```python
from build123d import *

# Parameters (mm, degrees)
F0_R     = 26
F0_R_2   = 14
F1_DEPTH = 12
F2_DEPTH = 178
F3_SIZE  = 2
F4_R     = 2.5
F5_DEPTH = 12
F7_DEPTH = 45
F8_R     = 5
F9_DEPTH = 22


with BuildPart() as f1:
    # F0 (on Right) → F1 (new body)
    with BuildSketch(Plane.YZ):
        Circle(F0_R)
        Circle(F0_R_2, mode=Mode.SUBTRACT)
        Circle(F0_R_2)
    extrude(amount=F1_DEPTH)

    # F0 (on Right) → F2 (join)
    with BuildSketch(Plane.YZ):
        Circle(F0_R_2)
    extrude(amount=F2_DEPTH)

    # F3
    f3_edges = [f1.edges().sort_by_distance(p)[0] for p in [
        (0, -26, 0),
        (178, -14, 0),
    ]]
    chamfer(f3_edges, length=F3_SIZE)

    # F4 (on face) → F5 (cut, through all)
    with BuildSketch(Plane(origin=(0, 0, 0), x_dir=(0, -1, 0), z_dir=(-1, 0, 0))):
        with Locations((21, 0)):
            Circle(F4_R)
    extrude(amount=-F5_DEPTH, mode=Mode.SUBTRACT)

    # F6 (on face) → F7 (cut)
    with BuildSketch(Plane.YZ.offset(178)):
        with BuildLine():
            Line((-11, 4.7958315233), (-11, 8.6602540378))
            ThreePointArc((-11, 8.6602540378), (-14, 0), (-11, -8.6602540378))
            Line((-11, -8.6602540378), (-11, -4.7958315233))
            ThreePointArc((-11, -4.7958315233), (-12, 0), (-11, 4.7958315233))
        make_face()
        with BuildLine():
            Line((-11, -4.7958315233), (-11, 4.7958315233))
            ThreePointArc((-11, 4.7958315233), (-12, 0), (-11, -4.7958315233))
        make_face()
        with BuildLine():
            ThreePointArc((12, 0), (11.7473401245, 2.4494897428), (11, 4.7958315233))
            Line((11, 4.7958315233), (11, -4.7958315233))
            ThreePointArc((11, -4.7958315233), (11.7473401245, -2.4494897428), (12, 0))
        make_face()
        with BuildLine():
            ThreePointArc((11, -8.6602540378), (13.2287565553, -4.582575695), (14, 0))
            ThreePointArc((14, 0), (13.2287565553, 4.582575695), (11, 8.6602540378))
            Line((11, 8.6602540378), (11, 4.7958315233))
            ThreePointArc((11, 4.7958315233), (11.7473401245, 2.4494897428), (12, 0))
            ThreePointArc((12, 0), (11.7473401245, -2.4494897428), (11, -4.7958315233))
            Line((11, -4.7958315233), (11, -8.6602540378))
        make_face()
    extrude(amount=-F7_DEPTH, mode=Mode.SUBTRACT)

    # F8 (on face) → F9 (cut, through all)
    with BuildSketch(Plane.XZ.offset(11)):
        with Locations((158, 0)):
            Circle(F8_R)
    extrude(amount=-F9_DEPTH, mode=Mode.SUBTRACT)


solid = f1.part
```
Source: CAD feature listing. Evaluate the final solid. Frame: model axes, mm. A direction names the side the tool comes from. Coordinates: 2 decimals unless noted, no trailing zeros. Loops run counter-clockwise (first coordinate to the right, second up) from the corner with the lowest first, then second, coordinate; pieces in that order, holes last. Notation, with made-up numbers: M 34,52 L 41,52 A34 ccw 41,88 Z; hole C 14.5,65 d7. An arc over 180 degrees is marked long. Use a Markdown table: item, result. Add a question column.
Q1. Material intervals for L1, parallel to X at y = -14.5, z = 16; L2, parallel to Z at x = 158, y = 5.25; L3, parallel to Y at x = 146, z = -1.5, sorted ascending.
Q2. Section query A-A, the plane x = 158. Return loops of the section in (y, z).
Q3. First-contact query: pin 1 (14 mm diameter, centred on x = 150, z = -2.5, fed in from +Y); pin 2 (2.5 mm diameter, centred on y = 13, z = 0, fed in from +X); pin 3 (4 mm diameter, centred on y = -2.5, z = -18, fed in from +X); pin 4 (8 mm diameter, centred on x = 158, z = 0, fed in from +Y). Flat tips, straight axial feed; report the tip coordinate or a pass-through.
Q4. Section query D-D, the plane x = 124.5. Return loops of the section in (y, z).
Q5. Section query B-B, the plane z = 0. Return loops of the section in (x, y).
Q6. Access query for faces 4 (the flat face through (151, -11, 0)), 5 (the flat face through (151, 11, 0)), 6 (the conical face through (0.125, -3.141, 23.92)), 7 (the flat face through (12, 11, -11)). Directions: +Z, -Z, +X, -X, +Y, -Y. A direction counts if a zero-diameter tool reaches every point of the face in a straight line with its end or side. Return the directions, or none.
Q7. Section query C-C, the plane y = 0. Return loops of the section in (x, z), and give its area (3 significant figures).
Q8. Draft query along Z for faces 1 (the flat face through (133, -12, 0)), 2 (the cylindrical face through (5.9, -18.5, 0.1)), 3 (the cylindrical face through (92.85, -1.82, 13.88)). Return one class per face: pulls with the +Z half, pulls with the -Z half, needs draft (parallel to the pull), parting line crosses it, or undercut.
Result:
| question | item | result |
|---|---|---|
| 1 | L1 | x = 0 to 12 |
| 1 | L2 | z = -12.98 to -5, 5 to 12.98 |
| 1 | L3 | y = -11 to 11 |
| 2 | outline | M -11,-8.66 A14 ccw 11,-8.66 L 11,-5 L -11,-5 Z; M -11,5 L 11,5 L 11,8.66 A14 ccw -11,8.66 Z |
| 3 | pin 1 | stops at y = 11 |
| 3 | pin 2 | stops at x = 133 |
| 3 | pin 3 | stops at x = 12 |
| 3 | pin 4 | passes through |
| 4 | outline | C 0,0 d28 |
| 5 | outline | M 0,-24 L 2,-26 L 12,-26 L 12,-23.5 L 0,-23.5 Z; M 0,-18.5 L 12,-18.5 L 12,-14 L 133,-14 L 133,-11 L 153,-11 L 153,11 L 133,11 L 133,14 L 12,14 L 12,26 L 2,26 L 0,24 Z; M 163,-11 L 178,-11 L 178,11 L 163,11 Z |
| 6 | face 4 | +Z, -Z, +X, -Y |
| 6 | face 5 | +Z, -Z, +X, +Y |
| 6 | face 6 | -X |
| 6 | face 7 | +X |
| 7 | outline | M 0,-24 L 2,-26 L 12,-26 L 12,-14 L 176,-14 L 178,-12 L 178,12 L 176,14 L 12,14 L 12,26 L 2,26 L 0,24 Z; hole C 158,0 d10 |
| 7 | area | 5,190 mm2 |
| 8 | face 1 | needs draft |
| 8 | face 2 | undercut |
| 8 | face 3 | parting line crosses it |
